```python
from build123d import *

# Parameters (mm, degrees)
SKETCH1_W                      = 120.65
SKETCH1_H                      = 40.64
BOSS_EXTRUDE1_DEPTH            = 1.5875
FILLET1_R                      = 6.35
SKETCH2_W                      = 40.64
SKETCH2_H                      = 19.05
BOSS_EXTRUDE2_DEPTH            = 31.75
FILLET2_R                      = 3.175
F_10_CLEARANCE_HOLE1_D         = 4.826
F_10_CLEARANCE_HOLE1_DEPTH     = 25.4
F_10_CLEARANCE_HOLE1_TIP       = 1.449876674
F_2_CLEARANCE_HOLE1_AT_2_COUNT = 2
F_2_CLEARANCE_HOLE1_AT_2_PITCH = 12.7
F_2_CLEARANCE_HOLE1_AT_3_COUNT = 2
F_2_CLEARANCE_HOLE1_AT_3_PITCH = 25.4
F_2_CLEARANCE_HOLE1_AT_4_COUNT = 2
F_2_CLEARANCE_HOLE1_AT_4_PITCH = 54.041188126
F_2_CLEARANCE_HOLE1_AT_5_COUNT = 2
F_2_CLEARANCE_HOLE1_AT_5_PITCH = 49.361726207
F_2_CLEARANCE_HOLE1_AT_6_COUNT = 2
F_2_CLEARANCE_HOLE1_AT_6_PITCH = 47.700000148
SKETCH13_R                     = 3.5749992
CUT_EXTRUDE1_DEPTH             = 72.856780691


with BuildPart() as part:
    # Sketch1 → Boss-Extrude1 (new body)
    with BuildSketch(Plane(origin=(0, 0, 0), x_dir=(1, 0, 0), z_dir=(0, 1, 0))):
        Rectangle(SKETCH1_W, SKETCH1_H)
    extrude(amount=BOSS_EXTRUDE1_DEPTH)

    # Fillet1
    fillet1_edges = [part.edges().sort_by_distance(p)[0] for p in [
        (60.325, 0.79375, 20.32),
        (-60.325, 0.79375, 20.32),
        (-60.325, 0.79375, -20.32),
        (60.325, 0.79375, -20.32),
    ]]
    fillet(fillet1_edges, radius=FILLET1_R)

    # Sketch2 → Boss-Extrude2 (add)
    with BuildSketch(Plane(origin=(0, 1.5875, 0), x_dir=(1, 0, 0), z_dir=(0, 1, 0))):
        Rectangle(SKETCH2_W, SKETCH2_H)
    extrude(amount=BOSS_EXTRUDE2_DEPTH)

    # Fillet2
    fillet2_edges = [part.edges().sort_by_distance(p)[0] for p in [
        (20.32, 17.4625, 9.525),
        (20.32, 17.4625, -9.525),
        (-20.32, 17.4625, -9.525),
        (-20.32, 17.4625, 9.525),
    ]]
    fillet(fillet2_edges, radius=FILLET2_R)

    # #10 Clearance Hole1
    with Locations(Plane(origin=(0, 33.3375, 0), x_dir=(1, 0, 0), z_dir=(0, 1, 0))):
        with Locations((-15.875, 0), (15.875, 0)):
            Hole(F_10_CLEARANCE_HOLE1_D / 2, depth=F_10_CLEARANCE_HOLE1_DEPTH)
            with Locations((0, 0, -(F_10_CLEARANCE_HOLE1_DEPTH + F_10_CLEARANCE_HOLE1_TIP / 2))):  # 118° drill point
                Cone(0, F_10_CLEARANCE_HOLE1_D / 2, F_10_CLEARANCE_HOLE1_TIP, mode=Mode.SUBTRACT)

    # Sketch12 → #2 Clearance Hole1 (revolve, cut)
    with BuildSketch(Plane(origin=(-23.850000074, 1.5875, -12.7), x_dir=(0, 0, 1), z_dir=(1, 0, 0))):
        Polygon((0, 0), (0, 1.5875), (1.0795, 1.5875), (1.0795, 0.827548112), (1.7145, 0), align=None)
    f_2_clearance_hole1 = revolve(axis=Axis((-23.850000074, 7.9375, -12.7), (0, -1, 0)), mode=Mode.SUBTRACT)

    # #2 Clearance Hole1 at 2: #2 Clearance Hole1 ×2
    with Locations(*[(0, 0, i * F_2_CLEARANCE_HOLE1_AT_2_PITCH) for i in range(1, F_2_CLEARANCE_HOLE1_AT_2_COUNT)]):
        add(f_2_clearance_hole1, mode=Mode.SUBTRACT)

    # #2 Clearance Hole1 at 3: #2 Clearance Hole1 ×2
    with Locations(*[(0, 0, i * F_2_CLEARANCE_HOLE1_AT_3_PITCH) for i in range(1, F_2_CLEARANCE_HOLE1_AT_3_COUNT)]):
        add(f_2_clearance_hole1, mode=Mode.SUBTRACT)

    # #2 Clearance Hole1 at 4: #2 Clearance Hole1 ×2
    with Locations(*[Vector(0.8826600931937462, 0, 0.4700118720662355) * (i * F_2_CLEARANCE_HOLE1_AT_4_PITCH) for i in range(1, F_2_CLEARANCE_HOLE1_AT_4_COUNT)]):
        add(f_2_clearance_hole1, mode=Mode.SUBTRACT)

    # #2 Clearance Hole1 at 5: #2 Clearance Hole1 ×2
    with Locations(*[Vector(0.9663357385056085, 0, 0.2572843572524773) * (i * F_2_CLEARANCE_HOLE1_AT_5_PITCH) for i in range(1, F_2_CLEARANCE_HOLE1_AT_5_COUNT)]):
        add(f_2_clearance_hole1, mode=Mode.SUBTRACT)

    # #2 Clearance Hole1 at 6: #2 Clearance Hole1 ×2
    with Locations(*[(i * F_2_CLEARANCE_HOLE1_AT_6_PITCH, 0, 0) for i in range(1, F_2_CLEARANCE_HOLE1_AT_6_COUNT)]):
        add(f_2_clearance_hole1, mode=Mode.SUBTRACT)

    # Sketch13 → Cut-Extrude1 (cut, through all)
    with BuildSketch(Plane(origin=(0, 0, 0), x_dir=(-1, 0, 0), z_dir=(0, -1, 0))):
        with Locations(Location((38.825000074, 0.042792778, 0), (0, 0, 90))):
            Circle(SKETCH13_R)
        with Locations(Location((-38.825000074, 0.042792778, 0), (0, 0, 270))):
            Circle(SKETCH13_R)
    extrude(amount=-CUT_EXTRUDE1_DEPTH, mode=Mode.SUBTRACT)


solid = part.part
```
Read the model definition and answer for the solid it produces. Units are mm, in the model's axes. A direction names the side the tool comes from. Give positions to 0.01 mm unless a question says otherwise; leave off trailing zeros. Write each loop counter-clockwise with the first axis right and the second up, starting at its lowest first coordinate (ties: lowest second). Pieces come first, ordered by that corner, then holes. Notation, with made-up numbers: (15, 70) - (19, 70) arc R28 cw to (19, 93) - close; hole circle Ø10 at (4, 81). An arc over 180 degrees is marked (long way). Write item = value, one per line. Start each with the question number.
Item 1: Find section A-A (z = -12.7). Give the vertices of the cut face in (x, y) (1 decimal), then the cut area to 3 significant figures.
Item 2: Each of these flat-tipped pins is pushed along its axis until it touches: P1, Ø2, axis at x = 20, z = 10, coming from the +Y side; P2, Ø4, axis at x = 15.875, z = 0, coming from the +Y side; P3, Ø1, axis at y = 25, z = 6, coming from the +X side; P4, Ø1.9, axis at x = -23.85, z = -12.7, coming from the +Y side. Where does it stop, or does it pass through?
Item 3: Find section D-D (x = 12). Give the vertices of the cut face in (y, z) (1 decimal).
Item 4: The mould has two halves that part along X. Classify faces 5 (the flat face through (0, 33.338, 0)), 6 (the cylindrical face through (58.514, 0.805, -18.41)), 7 (the cylindrical face through (24.808, 0.385, -12.202)): +X half, -X half, draft (parallel to the pull), parting line (faces both ways), or undercut.
Item 5: Find section C-C (y = 13). Give the vertices of the cut face in (x, z) (3 decimals).
Item 6: A tool of negligible diameter and unlimited length cuts with its end or side. For faces 1 (the cylindrical face through (-19.365, 17.685, -8.62)), 2 (the flat face through (-20.32, 17, 0)), 3 (the flat face through (20.32, 17, 0)), 4 (the flat face through (0, 17, -9.525)), from which of +Z, -Z, +X, -X, +Y, -Y can it reach the whole face along a straight path? Write none if from no direction.
Item 7: Find section B-B (x = -23.85). Give the vertices of the cut face in (y, z), then the cut area to 3 significant figures.
Item 8: Find the intervals of material crossed by probe 1 along Z at (x, y) = (-23.85, 0.5); probe 2 along X at (y, z) = (9, -0.5); probe 3 along Z at (x, y) = (-5, 13) (3 decimals), in increasing order. Write a range as [from, to].
Response:
q1.outline = (-60.3, 0) - (-24.9, 0) - (-24.9, 0.8) - (-25.6, 1.6) - (-60.3, 1.6) - close; (-22.8, 0) - (22.8, 0) - (22.8, 0.8) - (22.1, 1.6) - (-22.1, 1.6) - (-22.8, 0.8) - close; (24.9, 0) - (60.3, 0) - (60.3, 1.6) - (25.6, 1.6) - (24.9, 0.8) - close
q1.area = 184 mm²
q2.P1 = 1.59
q2.P2 = 7.69
q2.P3 = 20.32
q2.P4 = through
q3.outline = (0, -20.3) - (1.6, -20.3) - (1.6, -9.5) - (33.3, -9.5) - (33.3, 9.5) - (1.6, 9.5) - (1.6, 20.3) - (0, 20.3) - close
q4.face_5 = draft
q4.face_6 = +X half
q4.face_7 = undercut
q5.outline = (-20.32, -6.35) arc R3.175 ccw to (-17.145, -9.525) - (17.145, -9.525) arc R3.175 ccw to (20.32, -6.35) - (20.32, 6.35) arc R3.175 ccw to (17.145, 9.525) - (-17.145, 9.525) arc R3.175 ccw to (-20.32, 6.35) - close; hole circle Ø4.826 at (-15.875, 0); hole circle Ø4.826 at (15.875, 0)
q6.face_1 = -Z, -X, +Y
q6.face_2 = +Z, -Z, -X, +Y
q6.face_3 = +Z, -Z, +X, +Y
q6.face_4 = -Z, +X, -X, +Y
q7.outline = (0, -20.32) - (1.59, -20.32) - (1.59, -14.41) - (0.76, -13.78) - (0, -13.78) - close; (0, -11.62) - (0.76, -11.62) - (1.59, -10.99) - (1.59, -1.71) - (0.76, -1.08) - (0, -1.08) - close; (0, 1.08) - (0.76, 1.08) - (1.59, 1.71) - (1.59, 10.99) - (0.76, 11.62) - (0, 11.62) - close; (0, 13.78) - (0.76, 13.78) - (1.59, 14.41) - (1.59, 20.32) - (0, 20.32) - close
q7.area = 52.7 mm²
q8.probe_1 = [-20.32, -13.78], [-11.62, -1.08], [1.08, 11.62], [13.78, 20.32]
q8.probe_2 = [-20.32, -18.24], [-13.51, 13.51], [18.24, 20.32]
q8.probe_3 = [-9.525, 9.525]
